from build123d import *

# Parameters (mm, degrees)
F0_R     = 8.89
F1_DEPTH = 88.9
F4_DEPTH = 20.32
F6_DEPTH = 2.54


with BuildPart() as f1:
    # F0 (on Front) → F1 (new body)
    with BuildSketch(Plane.XZ):
        Circle(F0_R)
    extrude(amount=F1_DEPTH)

    # F2 (on face) → F4 (join)
    with BuildSketch(Plane.XZ.offset(88.9)):
        with BuildLine():
            ThreePointArc((-4.2918766229, -7.7853641568), (-7.6546353008, -4.5209134488), (-8.89, 0))
            Line((-8.89, 0), (-41.5729338972, -15.5504000302))
            Line((-41.5729338972, -15.5504000302), (-41.5729338972, -32.7917784452))
            Line((-41.5729338972, -32.7917784452), (-26.423625648, -32.7917784452))
            Line((-26.423625648, -32.7917784452), (-4.2918766229, -7.7853641568))
        make_face()
        with BuildLine():
            ThreePointArc((7.9221754919, -4.0337619507), (2.6102485031, -8.498158786), (-4.2918766229, -7.7853641568))
            Line((-4.2918766229, -7.7853641568), (7.6060682412, -32.7917784452))
            Line((7.6060682412, -32.7917784452), (24.2062564939, -40.108717978))
            Line((24.2062564939, -40.108717978), (31.0751149996, -24.5251063101))
            Line((31.0751149996, -24.5251063101), (7.9221754919, -4.0337619507))
        make_face()
        with BuildLine():
            Line((11.5068648519, 27.9272308745), (2.152897354, 8.6253772661))
            ThreePointArc((2.152897354, 8.6253772661), (5.536018968, 6.9559035348), (7.9221754919, 4.0337619507))
            Line((7.9221754919, 4.0337619507), (25.771754428, 17.6318820209))
            Line((25.771754428, 17.6318820209), (25.771754428, 34.7144042658))
            Line((25.771754428, 34.7144042658), (11.5068648519, 27.9272308745))
        make_face()
        with BuildLine():
            Line((-28.0105117708, 17.5770223141), (-5.7431249942, 6.7859130042))
            ThreePointArc((-5.7431249942, 6.7859130042), (-3.0582129907, 8.3474207576), (0, 8.89))
            Line((0, 8.89), (-12.7163026482, 32.8911244869))
            Line((-12.7163026482, 32.8911244869), (-28.0105117708, 32.8911244869))
            Line((-28.0105117708, 32.8911244869), (-28.0105117708, 17.5770223141))
        make_face()
        with BuildLine():
            ThreePointArc((-5.7431249942, 6.7859130042), (-8.0650009671, 3.7400346791), (-8.89, 0))
            ThreePointArc((-8.89, 0), (-7.6546353008, -4.5209134488), (-4.2918766229, -7.7853641568))
            ThreePointArc((-4.2918766229, -7.7853641568), (2.6102485031, -8.498158786), (7.9221754919, -4.0337619507))
            ThreePointArc((7.9221754919, -4.0337619507), (8.6446584699, -2.0741214859), (8.89, 0))
            ThreePointArc((8.89, 0), (8.6446584699, 2.0741214859), (7.9221754919, 4.0337619507))
            ThreePointArc((7.9221754919, 4.0337619507), (5.536018968, 6.9559035348), (2.152897354, 8.6253772661))
            ThreePointArc((2.152897354, 8.6253772661), (1.0845497001, 8.823596316), (0, 8.89))
            ThreePointArc((0, 8.89), (-3.0582129907, 8.3474207576), (-5.7431249942, 6.7859130042))
        make_face()
    extrude(amount=F4_DEPTH)

    # F5 (on face) → F6 (join)
    with BuildSketch(Plane.XZ.offset(109.22)):
        Polygon((7.6060682412, -32.7917784452), (15.9061623676, -36.4502482116), (20.813416993, -32.5923874103), (14.5969645539, -18.8207629411), align=None)
        Polygon((-4.2918766229, -7.7853641568), (1.6570958091, -20.288571301), (11.8639794051, -15.4321797825), align=None)
        Polygon((15.4445417704, -17.1269151278), (31.0751149996, -24.5251063101), (17.6763897155, -12.6666598402), align=None)
        Polygon((-26.423625648, -32.7917784452), (-14.1507707051, -9.8388109155), (-19.8614782116, -11.028258101), (-33.5180773118, -24.7176060956), align=None)
        Polygon((-19.7689795686, 25.8292742085), (0, 8.89), (-12.7163026482, 32.8911244869), align=None)
        Polygon((25.771754428, 34.7144042658), (7.9221754919, 4.0337619507), (25.771754428, 17.6318820209), align=None)
        Polygon((-41.5729338972, -32.7917784452), (-26.423625648, -32.7917784452), (-33.5180773118, -24.7176060956), align=None)
        Polygon((-28.0105117708, 17.5770223141), (0, 8.89), (-19.7689795686, 25.8292742085), align=None)
        Polygon((-41.5729338972, -15.5504000302), (-13.1555447136, -4.306243593), (-8.9251107789, -0.0656649632), (-8.89, 0), align=None)
    extrude(amount=F6_DEPTH)


solid = f1.part
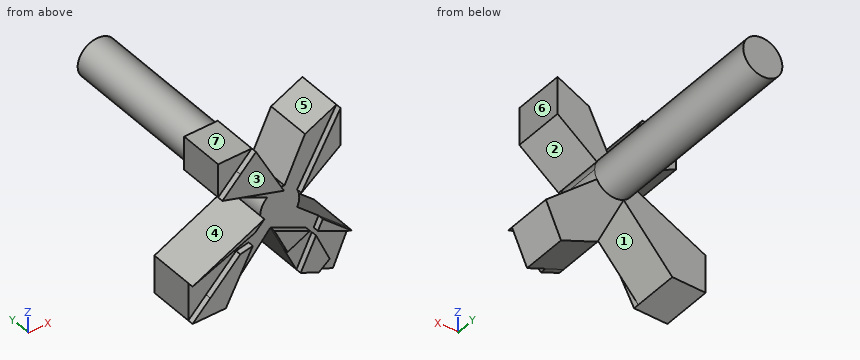
Geometry: final body of the model. Coordinates: model frame, mm. Face numbers are marked on the shaded views. A direction names the side the tool comes from. Give positions to 0.01 mm unless a question says otherwise; leave off trailing zeros. Loops run counter-clockwise (first coordinate to the right, second up) from the corner with the lowest first, then second, coordinate; pieces in that order, holes last. Notation, with made-up numbers: (58, 35.25) - (71, 35.25) arc R16 ccw to (71, 47.25) - close; hole circle Ø1 at (82, 43.25). An arc over 180 degrees is marked (long way). Answer as CSV lines item,"result". Start each with the question number.
1. Section C-C, the plane x = -36.5. Return loops of the section in (y, z), plus the area to 3 significant figures.
2. Pin query (flat end, axial travel): P1, Ø17.5, axis at x = 9, z = -22.5, coming from the +Y side; P2, Ø12, axis at x = -37.5, y = -103, coming from the -Z side; P3, Ø4, axis at y = -94.5, z = 14.5, coming from the +X side. Return the tip coordinate at first contact, or that it passes through.
3. Reachability of the marked faces 5, 6 and 7 from +Z, -Z, +X, -X, +Y, -Y: full face, straight path, thin tool, end or side. Return the list, or none.
4. Section A-A, the plane z = -14. Return loops of the section in (x, y), plus the area to 3 significant figures.
5. Section B-B, the plane y = -101.5. Return loops of the section in (x, z), plus the area to 3 significant figures.
6. Section D-D, the plane z = 14. Return loops of the section in (x, y).
7. Draft query along Z for the marked faces 1, 2, 3 and 4. Return one class per face: released by +Z, released by -Z, zero draft, split by the parting line, or undercut.
8. Ray query, L1, parallel to Y at x = -5, z = 15; L2, parallel to Z at x = -26, y = -93; L3, parallel to Z at x = 11, y = -93. Return the intervals inside material, ascending.
Answers:
1,outline,"(-111.76, -32.79) - (-88.9, -32.79) - (-88.9, -13.14) - (-111.76, -13.14) - (-111.76, -13.54) - (-109.22, -13.54) - (-109.22, -27.71) - (-111.76, -27.71) - close"
1,area,"413 mm2"
2,P1,"stops at y = -88.9"
2,P2,"stops at z = -32.79"
2,P3,"stops at x = 24.29"
3,face 5,"+Z, +Y, -Y"
3,face 6,"+Z, +X, +Y, -Y"
3,face 7,"+Z, -X, +Y, -Y"
4,outline,"(-38.31, -111.76) - (-37.65, -111.76) - (-37.65, -109.22) - (-22.83, -109.22) - (-22.83, -111.76) - (-16.38, -111.76) - (-16.38, -109.22) - (-9.79, -109.22) - (-9.79, -88.9) - (-38.31, -88.9) - close; (-1.33, -111.76) - (8.84, -111.76) - (8.84, -109.22) - (17.01, -109.22) - (17.01, -111.76) - (19.18, -111.76) - (19.18, -88.9) - (-1.33, -88.9) - close"
4,area,"1,050 mm2"
5,outline,"(-41.57, -32.79) - (-26.42, -32.79) - (-4.29, -7.79) - (7.61, -32.79) - (24.21, -40.11) - (31.08, -24.53) - (7.92, -4.03) arc R8.89 ccw to (7.92, 4.03) - (25.77, 17.63) - (25.77, 34.71) - (11.51, 27.93) - (2.15, 8.63) arc R8.89 ccw to (0, 8.89) - (-12.72, 32.89) - (-28.01, 32.89) - (-28.01, 17.58) - (-5.74, 6.79) arc R8.89 ccw to (-8.89, 0) - (-41.57, -15.55) - close"
5,area,"2,390 mm2"
6,outline,"(-20.63, -109.22) - (-16.48, -109.22) - (-16.48, -111.76) - (-2.71, -111.76) - (-2.71, -88.9) - (-20.63, -88.9) - close; (4.76, -109.22) - (13.72, -109.22) - (13.72, -111.76) - (21, -111.76) - (21, -88.9) - (4.76, -88.9) - close"
7,face 1,"released by -Z"
7,face 2,"undercut"
7,face 3,"zero draft"
7,face 4,"undercut"
8,L1,"y = -111.76 to -88.9"
8,L2,"z = -32.31 to -8.14, 16.6 to 32.89"
8,L3,"z = -34.29 to -6.76, 6.38 to 26.88"
